Check sheet for the modelled part. Datum: model origin and axes. Units: mm. Give positions to 0.01 mm unless a question says otherwise; leave off trailing zeros. Write each loop counter-clockwise with the first axis right and the second up, starting at its lowest first coordinate (ties: lowest second). Pieces come first, ordered by that corner, then holes. Notation, with made-up numbers: (39, -39.75) -> (61, -39.75) arc R18 ccw to (61, -32.75) -> close; hole circle Ø2 at (-24.75, 28). An arc over 180 degrees is marked (long way). Return JSON: item names as keys, results as strings.
from build123d import *

# Parameters (mm, degrees)
SKETCH1_R              = 2.2479
BOSS_EXTRUDE1_DEPTH    = 3.175
STAND_OFF_THRU_HOLES_D = 10.0838
SENSOR_THRU_HOLES_D    = 11


with BuildPart() as part:
    # Sketch1 → Boss-Extrude1 (new body)
    with BuildSketch(Plane.XY):
        with BuildLine():
            ThreePointArc((115.886477974, -22.233403312), (0, 118), (-115.886477974, -22.233403312))
            ThreePointArc((-115.886477974, -22.233403312), (0, -118), (115.886477974, -22.233403312))
        make_face()
        with Locations((109.1, 0)):
            Circle(SKETCH1_R, mode=Mode.SUBTRACT)
        with Locations((106.71590324, -22.683165468)):
            Circle(SKETCH1_R, mode=Mode.SUBTRACT)
        with Locations((99.667809429, -44.37496776)):
            Circle(SKETCH1_R, mode=Mode.SUBTRACT)
        with Locations((88.263754086, -64.127371025)):
            Circle(SKETCH1_R, mode=Mode.SUBTRACT)
        with Locations((73.002149154, -81.07710046)):
            Circle(SKETCH1_R, mode=Mode.SUBTRACT)
        with Locations((54.55, -94.483371553)):
            Circle(SKETCH1_R, mode=Mode.SUBTRACT)
        with Locations((33.713754086, -103.760265928)):
            Circle(SKETCH1_R, mode=Mode.SUBTRACT)
        with Locations((11.404055343, -108.502338785)):
            Circle(SKETCH1_R, mode=Mode.SUBTRACT)
        with Locations((-11.404055343, -108.502338785)):
            Circle(SKETCH1_R, mode=Mode.SUBTRACT)
        with Locations((-33.713754086, -103.760265928)):
            Circle(SKETCH1_R, mode=Mode.SUBTRACT)
        with Locations((-54.55, -94.483371553)):
            Circle(SKETCH1_R, mode=Mode.SUBTRACT)
        with Locations((-73.002149154, -81.07710046)):
            Circle(SKETCH1_R, mode=Mode.SUBTRACT)
        with Locations((-88.263754086, -64.127371025)):
            Circle(SKETCH1_R, mode=Mode.SUBTRACT)
        with Locations((-99.667809429, -44.37496776)):
            Circle(SKETCH1_R, mode=Mode.SUBTRACT)
        with Locations((-106.71590324, -22.683165468)):
            Circle(SKETCH1_R, mode=Mode.SUBTRACT)
        with Locations((-109.1, 0)):
            Circle(SKETCH1_R, mode=Mode.SUBTRACT)
        with Locations((-106.71590324, 22.683165468)):
            Circle(SKETCH1_R, mode=Mode.SUBTRACT)
        with Locations((-99.667809429, 44.37496776)):
            Circle(SKETCH1_R, mode=Mode.SUBTRACT)
        with Locations((-88.263754086, 64.127371025)):
            Circle(SKETCH1_R, mode=Mode.SUBTRACT)
        with Locations((-73.002149154, 81.07710046)):
            Circle(SKETCH1_R, mode=Mode.SUBTRACT)
        with Locations((-54.55, 94.483371553)):
            Circle(SKETCH1_R, mode=Mode.SUBTRACT)
        with Locations((-33.713754086, 103.760265928)):
            Circle(SKETCH1_R, mode=Mode.SUBTRACT)
        with Locations((-11.404055343, 108.502338785)):
            Circle(SKETCH1_R, mode=Mode.SUBTRACT)
        with Locations((11.404055343, 108.502338785)):
            Circle(SKETCH1_R, mode=Mode.SUBTRACT)
        with Locations((33.713754086, 103.760265928)):
            Circle(SKETCH1_R, mode=Mode.SUBTRACT)
        with Locations((54.55, 94.483371553)):
            Circle(SKETCH1_R, mode=Mode.SUBTRACT)
        with Locations((73.002149154, 81.07710046)):
            Circle(SKETCH1_R, mode=Mode.SUBTRACT)
        with Locations((88.263754086, 64.127371025)):
            Circle(SKETCH1_R, mode=Mode.SUBTRACT)
        with Locations((99.667809429, 44.37496776)):
            Circle(SKETCH1_R, mode=Mode.SUBTRACT)
        with Locations((106.71590324, 22.683165468)):
            Circle(SKETCH1_R, mode=Mode.SUBTRACT)
    extrude(amount=BOSS_EXTRUDE1_DEPTH)

    # Stand-off Thru Holes (through all)
    with Locations(Plane(origin=(0, 0, 0), x_dir=(-1, 0, 0), z_dir=(0, 0, -1))):
        with Locations((50, -37.5), (50, 37.5), (-50, 37.5), (-50, -37.5)):
            Hole(STAND_OFF_THRU_HOLES_D / 2)

    # Sensor Thru Holes (through all)
    with Locations(Plane(origin=(20, 70, 0), x_dir=(-1, 0, 0), z_dir=(0, 0, -1))):
        with Locations((0, 0), (40, 0)):
            Hole(SENSOR_THRU_HOLES_D / 2)


solid = part.part
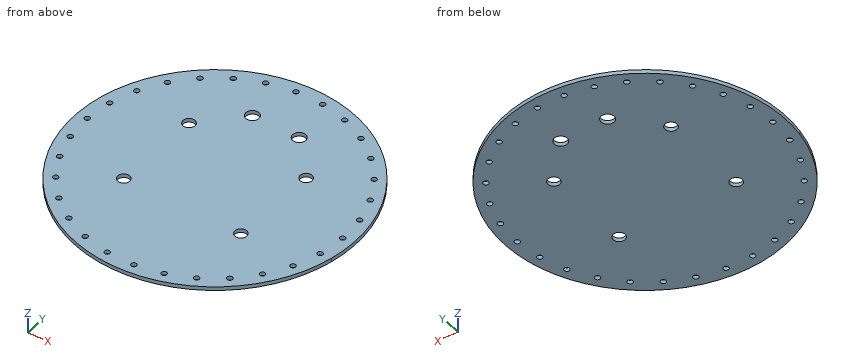
(1) Cross-section at A-A on x = -20. Enter the section's corners in (y, z) (3 decimals), then the cut area to 3 significant figures.
Reply:
{"outline": "(-116.293, 0) -> (64.5, 0) -> (64.5, 3.175) -> (-116.293, 3.175) -> close; (75.5, 0) -> (116.293, 0) -> (116.293, 3.175) -> (75.5, 3.175) -> close", "area": "704 mm^2"}
(2) Depth check by flat-ended pin: pin 1 Ø1 at (y, z) = (-57.5, 1) entering from -X; pin 2 Ø1 at (y, z) = (30.5, 3) entering from +X. Enter the tip coordinate at first touch or a pass-through.
Reply:
{"pin 1": "x = -103.32", "pin 2": "x = 114.12"}
(3) Thickness scan on L1, parallel to X at y = -80, z = 0.55; L2, parallel to X at y = 96, z = 2.8; L3, parallel to X at y = -59.5, z = 2.85. Record the ranges inside material, lowest first.
Reply:
{"L1": "-86.74 to -74.98, -71.03 to 71.03, 74.98 to 86.74", "L2": "-68.61 to -56.21, -52.89 to 52.89, 56.21 to 68.61", "L3": "-101.9 to 101.9"}
(4) Cross-section at C-C on z = 2.1. State how many separate pieces and enclosed holes the cut face has, then the cut area to 3 significant figures.
Reply:
{"separate pieces": "1", "enclosed holes": "36", "area": "42,800 mm^2"}
(5) Cross-section at B-B on y = 37.5. Enter the section's corners in (x, z) (3 decimals).
Reply:
{"outline": "(-111.883, 0) -> (-55.042, 0) -> (-55.042, 3.175) -> (-111.883, 3.175) -> close; (-44.958, 0) -> (44.958, 0) -> (44.958, 3.175) -> (-44.958, 3.175) -> close; (55.042, 0) -> (111.883, 0) -> (111.883, 3.175) -> (55.042, 3.175) -> close"}
